Design review of the part shown in the three views and the two pictorial views. Dimensions are in mm from the part's minimum x, y and z. A direction names the side the tool comes from. Coordinates: 2 decimals unless noted, no trailing zeros. Loops run counter-clockwise (first coordinate to the right, second up) from the corner with the lowest first, then second, coordinate; pieces in that order, holes last.
Q1. Add section C-C on z = 3.25. Give the boundary of the cut face in (x, y).
Q2. Wall thickness on probe 1 along Z at (x, y) = (16, 24); probe 2 along Y at (x, z) = (12.5, 6.75); probe 3 along Y at (x, z) = (12.5, 22.25): over which ranges is each line inside the solid? List them lowest first.
Q3. Machinability: for the marked faces 1, 2 and 3, which of the approach directions +Z, -Z, +X, -X, +Y, -Y give a long, thin tool a straight path to every point of the face, cutting with its end or side? Answer none if there is none.
Q4. Add section B-B on y = 14. Give the boundary of the cut face in (x, z), and give its area (3 significant figures).
Q5. Add section D-D on x = 21. Give the boundary of the cut face in (y, z), and give its area (3 significant figures).
Q6. For P1, Ø2, axis at x = 15.5, z = 15.5, coming from the +Y side; P2, Ø8, axis at y = 20, z = 4, coming from the -X side; P3, Ø6, axis at y = 6, z = 9.5, coming from the -X side, all flat-tipped, find the tip position at first contact; note any pin that passes through.
Q7. Add section A-A on x = 12.5. Give the boundary of the cut face in (y, z).
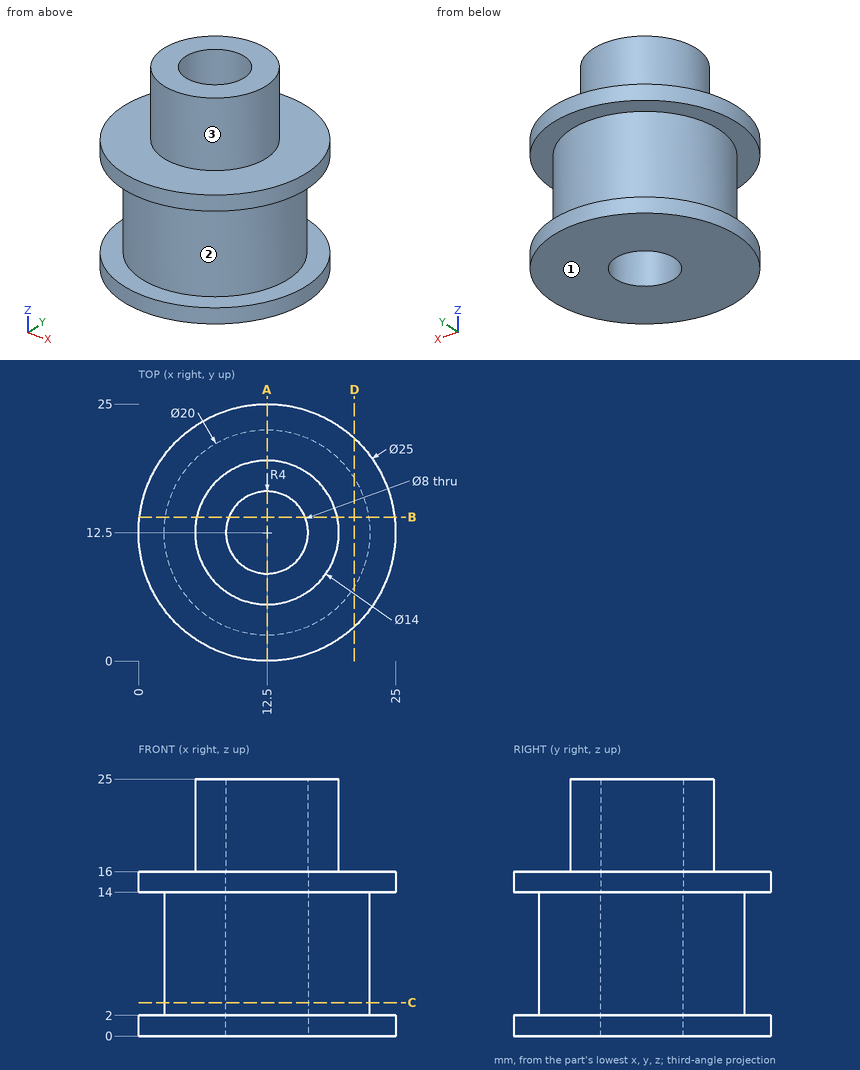
Entries:
1. outline: circle Ø20 at (12.5, 12.5); hole circle Ø8 at (12.5, 12.5)
2. probe 1: z = 0 to 2, 14 to 16
2. probe 2: y = 2.5 to 8.5, 16.5 to 22.5
2. probe 3: y = 5.5 to 8.5, 16.5 to 19.5
3. face 1: -Z, +X, -X, +Y, -Y
3. face 2: none
3. face 3: +Z
4. outline: (0.09, 0) - (8.79, 0) - (8.79, 25) - (5.66, 25) - (5.66, 16) - (0.09, 16) - (0.09, 14) - (2.61, 14) - (2.61, 2) - (0.09, 2) - close; (16.21, 0) - (24.91, 0) - (24.91, 2) - (22.39, 2) - (22.39, 14) - (24.91, 14) - (24.91, 16) - (19.34, 16) - (19.34, 25) - (16.21, 25) - close
4. area: 274 mm2
5. outline: (3.33, 0) - (21.67, 0) - (21.67, 2) - (17.77, 2) - (17.77, 14) - (21.67, 14) - (21.67, 16) - (3.33, 16) - (3.33, 14) - (7.23, 14) - (7.23, 2) - (3.33, 2) - close
5. area: 200 mm2
6. P1: stops at y = 24.84
6. P2: stops at x = 0.67
6. P3: stops at x = 3.13
7. outline: (0, 0) - (8.5, 0) - (8.5, 25) - (5.5, 25) - (5.5, 16) - (0, 16) - (0, 14) - (2.5, 14) - (2.5, 2) - (0, 2) - close; (16.5, 0) - (25, 0) - (25, 2) - (22.5, 2) - (22.5, 14) - (25, 14) - (25, 16) - (19.5, 16) - (19.5, 25) - (16.5, 25) - close
